Autodesk Inventor part; units mm, degrees
ref_plane "YZ Plane" through (0, 0, 0) normal (1, 0, 0) x (0, 1, 0)
ref_plane "XZ Plane" through (0, 0, 0) normal (0, 1, 0) x (-1, 0, 0)
ref_plane "XY Plane" through (0, 0, 0) normal (0, 0, 1) x (1, 0, 0)
sketch "草图1" plane through (0, 0, 0) normal (0, 0, 1) x (1, 0, 0)
  circle A0 centre (0, 0) radius 225
  dimension "d0" = 450
surface extrude "拉伸曲面1" sketch "草图1" along normal blind 700 shown no curves A0
thicken "加厚1" operation new thickness 3.7 both sides no extend neighbours no toward (-0.9057566, 0.4237984, 0) faces at (203.7952, -95.3546, 466.6667)
sketch "草图2" plane through (0, 0, 700) normal (0, 0, 1) x (1, 0, 0)
  circle A0 centre (0, 0) radius 225
  circle A1 centre (0, 0) radius 221.3
  circle A2 centre (0, 0) radius 290
  dimension "d18" = 580
  dimension "d19" = 442.6
  dimension "d20" = 450
extrude "拉伸1" add sketch "草图2" against normal blind 15 contours A2
sketch "草图3" plane through (0, 0, 700) normal (0, 0, 1) x (1, 0, 0)
  circle A0 centre (0, 0) radius 290
  circle A1 centre (0, 0) radius 221.3
  line L0 (0, -221.3) -> (0, -290)
  point P0 (0, -255.65)
  point P1 (180.7718, -180.7718)
  point P2 (255.65, 0)
  point P3 (180.7718, 180.7718)
  point P4 (0, 255.65)
  point P5 (-180.7718, 180.7718)
  point P6 (-255.65, 0)
  point P7 (-180.7718, -180.7718)
  dimension "d9" = 360
  dimension "d21" = 255.65
hole "孔1" at (0, -255.65, 700) at (180.7718, -180.7718, 700) at (255.65, 0, 700) at (180.7718, 180.7718, 700) at (0, 255.65, 700) at (-180.7718, 180.7718, 700) at (-255.65, 0, 700) at (-180.7718, -180.7718, 700) direction (0, 0, -1) diameter 20 end through all
sketch "草图4" plane through (0, 0, 0) normal (1, 0, 0) x (0, 1, 0)
  line L0 (-225, 685) -> (225, 685)
  line L1 (225, 0) -> (-225, 0)
  line L2 (225, 0) -> (-225, 0)
  line L3 (-225, 0) -> (225, 342.5)
  line L4 (225, 0) -> (225, 685)
  point P0 (0, 0)
extrude "拉伸2" cut sketch "草图4" along normal mid plane 1000
properties part number "进气孔"
Input: part model. Units: mm. Frame: model coordinates. Give positions to 0.01 mm unless a question says otherwise; leave off trailing zeros. Order: outer loops, then holes, each group sorted by start corner. A loop starts at its lowest first (then second) coordinate and runs counter-clockwise, first axis right, second up. Notation, with made-up numbers: (42, -22.5) - (54, -22.5) arc R18 cw to (54, -1.5) - close; hole circle Ø10 at (79, -35). An arc over 180 degrees is marked (long way). Put each result on its own line as item: value.
Item 1: Section query D-D, the plane z = 439.5. Return loops of the section in (x, y).
Found:
outline: circle Ø450 at (0, 0); hole circle Ø442.6 at (0, 0)
Item 2: Contact query for flat-ended pins moving along their axis: pin 1 (1 mm diameter, centred on y = -56, z = 217.5, fed in from +X); pin 2 (3 mm diameter, centred on y = -48.5, z = 376, fed in from -X); pin 3 (1 mm diameter, centred on x = 94.5, z = 198.5, fed in from -Y); pin 4 (16 mm diameter, centred on x = 0, y = 255.65, fed in from -Z). Output: stop coordinate, or through.
Found:
pin 1: stops at x = 218.05
pin 2: stops at x = -220.04
pin 3: stops at y = -204.42
pin 4: passes through
Item 3: Section query B-B, the plane x = 0. Return loops of the section in (y, z).
Found:
outline: (-290, 685) - (-265.65, 685) - (-265.65, 700) - (-290, 700) - close; (-245.65, 685) - (-225, 685) - (-225, 0) - (-221.3, 2.82) - (-221.3, 700) - (-245.65, 700) - close; (221.3, 339.68) - (225, 342.5) - (225, 685) - (245.65, 685) - (245.65, 700) - (221.3, 700) - close; (265.65, 685) - (290, 685) - (290, 700) - (265.65, 700) - close
Item 4: Section query C-C, the plane y = 98. Return loops of the section in (x, z), then the cut area to 3 significant figures.
Found:
outline: (-272.94, 685) - (-202.54, 685) - (-202.54, 245.84) - (-198.42, 245.84) - (-198.42, 700) - (-272.94, 700) - close; (198.42, 245.84) - (202.54, 245.84) - (202.54, 685) - (272.94, 685) - (272.94, 700) - (198.42, 700) - close
area: 5,850 mm^2
Item 5: Draft query along X for faces 1 (the cylindrical face through (-29.291, -223.085, 413.814)), 2 (the flat face through (-216, 66, 685)), 3 (the cylindrical face through (-28.809, -219.417, 423.768)). Return one class per face: +X half, -X half, draft (parallel to the pull), parting line (faces both ways), or undercut.
Found:
face 1: parting line
face 2: draft
face 3: undercut
Item 6: Ray query, L1, parallel to Y at x = 0, z = 688.75; L2, parallel to X at y = 0, z = 560; L3, parallel to Z at x = 120, y = -256.5. Return the intervals inside material, ascending. Write a range as from..to.
Found:
L1: y = -290..-265.65, -245.65..-221.3, 221.3..245.65, 265.65..290
L2: x = -225..-221.3, 221.3..225
L3: z = 685..700
Item 7: Section query A-A, the plane y = 0. Return loops of the section in (x, z), then the cut area to 3 significant figures.
Found:
outline: (-290, 685) - (-265.65, 685) - (-265.65, 700) - (-290, 700) - close; (-245.65, 685) - (-225, 685) - (-225, 171.25) - (-221.3, 171.25) - (-221.3, 700) - (-245.65, 700) - close; (221.3, 171.25) - (225, 171.25) - (225, 685) - (245.65, 685) - (245.65, 700) - (221.3, 700) - close; (265.65, 685) - (290, 685) - (290, 700) - (265.65, 700) - close
area: 5,260 mm^2
